Source: three-view drawing plus pictorial views. Frame: mm from the lowest corner of the part. Round coordinates to 2 decimals unless told otherwise and drop trailing zeros. Loops run counter-clockwise (first coordinate to the right, second up) from the corner with the lowest first, then second, coordinate; pieces in that order, holes last. Notation, with made-up numbers: M 11.25,46.5 L 57.25,46.5 A27 cw 57.25,72.5 Z; hole C 8.5,53.5 d10. An arc over 180 degrees is marked long. Return JSON: item names as keys, results as strings. Group by question number.
1) Section C-C (z = 6.35). Output: boundary loops of the cut face in (x, y).
2) Material intervals for line 1 (X direction, y = 44.5, z = 6.35); line 2 (X direction, y = 41.5, z = 9); line 3 (X direction, y = 35, z = 1), sorted ascending. Write a range as from..to.
3) Section D-D (z = 11.5). Output: boundary loops of the cut face in (x, y), plus the area to 3 significant figures.
4) Section B-B (y = 36). Output: boundary loops of the cut face in (x, z) (1 decimal).
5) Section A-A (x = 7.62). Output: boundary loops of the cut face in (y, z).
6) Contact query for flat-ended pins moving along their axis: P1, Ø6, axis at y = 5.5, z = 2.5, coming from the -X side (1 decimal); P2, Ø2, axis at y = 28.5, z = 9.5, coming from the +X side; P3, Ø4, axis at x = 101, z = 2.5, coming from the -Y side. Output: stop coordinate, or through.
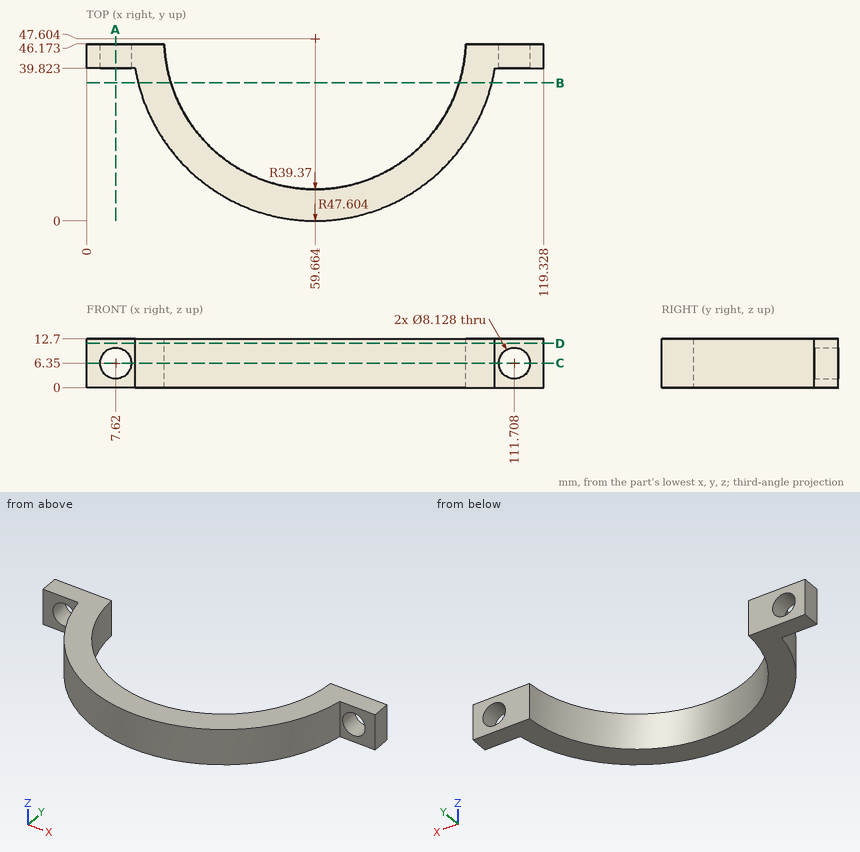
Returned:
{
 "1": {"outline": "M 0,39.82 L 3.56,39.82 L 3.56,46.17 L 0,46.17 Z; M 11.68,39.82 L 12.7,39.82 A47.6 ccw 106.63,39.82 L 107.64,39.82 L 107.64,46.17 L 99.01,46.17 A39.37 cw 20.32,46.17 L 11.68,46.17 Z; M 115.77,39.82 L 119.33,39.82 L 119.33,46.17 L 115.77,46.17 Z"},
 "2": {"line 1": "x = 0..3.56, 11.68..20.42, 98.91..107.64, 115.77..119.33", "line 2": "x = 0..4.54, 10.7..20.77, 98.56..108.63, 114.79..119.33", "line 3": "x = 13.76..22.37, 96.96..105.57"},
 "3": {"outline": "M 0,39.82 L 12.7,39.82 A47.6 ccw 106.63,39.82 L 119.33,39.82 L 119.33,46.17 L 99.01,46.17 A39.37 cw 20.32,46.17 L 0,46.17 Z", "area": "1,260 mm^2"},
 "4": {"outline": "M 13.5,0 L 22,0 L 22,12.7 L 13.5,12.7 Z; M 97.3,0 L 105.8,0 L 105.8,12.7 L 97.3,12.7 Z"},
 "5": {"outline": "M 39.82,0 L 46.17,0 L 46.17,2.29 L 39.82,2.29 Z; M 39.82,10.41 L 46.17,10.41 L 46.17,12.7 L 39.82,12.7 Z"},
 "6": {"P1": "stops at x = 32.5", "P2": "stops at x = 103.69", "P3": "stops at y = 20.79"}
}
